Work out the finished part from the listing and answer in its coordinate system (mm). A direction names the side the tool comes from. Round coordinates to 2 decimals unless told otherwise and drop trailing zeros. Loops run counter-clockwise (first coordinate to the right, second up) from the corner with the lowest first, then second, coordinate; pieces in that order, holes last. Notation, with made-up numbers: (81.25, 74) -> (121.25, 74) arc R19 cw to (121.25, 82) -> close; hole circle Ø6 at (-2.5, 22). An arc over 180 degrees is marked (long way). Use one line per item in the form item = value.
```python
from build123d import *

# Parameters (mm, degrees)
BOSS_EXTRUDE1_DEPTH = 2
SKETCH2_W           = 40.18
SKETCH2_H           = 12.8
CUT_EXTRUDE1_DEPTH  = 1
SKETCH3_W           = 38.18
SKETCH3_H           = 10.8
CUT_EXTRUDE4_DEPTH  = 3
SKETCH4_W           = 2
SKETCH4_H           = 2
CUT_EXTRUDE5_DEPTH  = 3
SKETCH5_R           = 4
CUT_EXTRUDE6_DEPTH  = 5
SKETCH7_W           = 40.18
SKETCH7_H           = 2
BOSS_EXTRUDE2_DEPTH = 5
CUT_EXTRUDE10_DEPTH = 1
SKETCH12_W          = 40
SKETCH12_H          = 40
CUT_EXTRUDE11_DEPTH = 1
CUT_EXTRUDE12_REACH = 8
SKETCH13_R          = 1.75


with BuildPart() as part:
    # Sketch1 → Boss-Extrude1 (new body)
    with BuildSketch(Plane.XY):
        with BuildLine():
            Line((-70, -63.636363636), (70, -63.636363636))
            ThreePointArc((70, -63.636363636), (92.201532545, -2.475903873), (40, 36.363636364))
            Line((40, 36.363636364), (-40, 36.363636364))
            ThreePointArc((-40, 36.363636364), (-92.201532545, -2.475903873), (-70, -63.636363636))
        make_face()
    extrude(amount=BOSS_EXTRUDE1_DEPTH)

    # Sketch2 → Cut-Extrude1 (cut)
    with BuildSketch(Plane.XY):
        with Locations((0, 14.564946817)):
            Rectangle(SKETCH2_W, SKETCH2_H)
    extrude(amount=CUT_EXTRUDE1_DEPTH, mode=Mode.SUBTRACT)

    # Sketch3 → Cut-Extrude4 (cut, through all)
    with BuildSketch(Plane.XY):
        with Locations((0, 14.564946817)):
            Rectangle(SKETCH3_W, SKETCH3_H)
    extrude(amount=CUT_EXTRUDE4_DEPTH, mode=Mode.SUBTRACT)

    # Sketch4 → Cut-Extrude5 (cut, through all)
    with BuildSketch(Plane.XY.offset(2)):
        with Locations((-39, 35.363636364)):
            Rectangle(SKETCH4_W, SKETCH4_H)
        with Locations((39, 35.363636364)):
            Rectangle(SKETCH4_W, SKETCH4_H)
        with Locations((-68.39388, -62.636363636)):
            Rectangle(SKETCH4_W, SKETCH4_H)
        with Locations((68.39388, -62.636363636)):
            Rectangle(SKETCH4_W, SKETCH4_H)
    extrude(amount=-CUT_EXTRUDE5_DEPTH, mode=Mode.SUBTRACT)

    # Sketch5 → Cut-Extrude6 (cut)
    with BuildSketch(Plane.XY):
        with Locations((0, -15.909090909)):
            Circle(SKETCH5_R)
        with Locations((0, -39.772727273)):
            Circle(SKETCH5_R)
        with Locations((25, -39.772727273)):
            Circle(SKETCH5_R)
        with Locations((50, -39.772727273)):
            Circle(SKETCH5_R)
        with Locations((-25, -39.772727273)):
            Circle(SKETCH5_R)
        with Locations((-50, -39.772727273)):
            Circle(SKETCH5_R)
    extrude(amount=CUT_EXTRUDE6_DEPTH, mode=Mode.SUBTRACT)

    # Sketch7 → Boss-Extrude2 (add)
    with BuildSketch(Plane(origin=(0, 0, 0), x_dir=(-1, 0, 0), z_dir=(0, 0, -1))):
        with Locations((0, 7.164946817)):
            Rectangle(SKETCH7_W, SKETCH7_H)
    extrude(amount=BOSS_EXTRUDE2_DEPTH)

    # Sketch11 → Cut-Extrude10 (cut)
    with BuildSketch(Plane(origin=(0, 0, 0), x_dir=(-1, 0, 0), z_dir=(0, 0, -1))):
        Polygon((-60, -29.772727273), (-10, -29.772727273), (-10, -5.909090909), (10, -5.909090909), (10, -29.772727273), (60, -29.772727273), (60, -49.772727273), (-60, -49.772727273), align=None)
    extrude(amount=-CUT_EXTRUDE10_DEPTH, mode=Mode.SUBTRACT)

    # Sketch12 → Cut-Extrude11 (cut)
    with BuildSketch(Plane.XY.offset(2)):
        with Locations((50, -4.772727273)):
            Rectangle(SKETCH12_W, SKETCH12_H)
    extrude(amount=-CUT_EXTRUDE11_DEPTH, mode=Mode.SUBTRACT)

    # Sketch13 → Cut-Extrude12 (cut, up to next)
    with BuildSketch(Plane.XY.offset(1), mode=Mode.PRIVATE) as cut_extrude12_sk1:
        with Locations((33, 12.227272727)):
            Circle(SKETCH13_R)
    cut_extrude12_tool1 = extrude(cut_extrude12_sk1.sketch, amount=-CUT_EXTRUDE12_REACH, mode=Mode.PRIVATE) & part.part
    add(cut_extrude12_tool1.solids().sort_by_distance((33, 12.227273, 1))[0], mode=Mode.SUBTRACT)
    # Sketch13 → Cut-Extrude12 (cut, up to next)
    with BuildSketch(Plane.XY.offset(1), mode=Mode.PRIVATE) as cut_extrude12_sk2:
        with Locations((67, 12.227272727)):
            Circle(SKETCH13_R)
    cut_extrude12_tool2 = extrude(cut_extrude12_sk2.sketch, amount=-CUT_EXTRUDE12_REACH, mode=Mode.PRIVATE) & part.part
    add(cut_extrude12_tool2.solids().sort_by_distance((67, 12.227273, 1))[0], mode=Mode.SUBTRACT)
    # Sketch13 → Cut-Extrude12 (cut, up to next)
    with BuildSketch(Plane.XY.offset(1), mode=Mode.PRIVATE) as cut_extrude12_sk3:
        with Locations((33, -21.772727273)):
            Circle(SKETCH13_R)
    cut_extrude12_tool3 = extrude(cut_extrude12_sk3.sketch, amount=-CUT_EXTRUDE12_REACH, mode=Mode.PRIVATE) & part.part
    add(cut_extrude12_tool3.solids().sort_by_distance((33, -21.772727, 1))[0], mode=Mode.SUBTRACT)
    # Sketch13 → Cut-Extrude12 (cut, up to next)
    with BuildSketch(Plane.XY.offset(1), mode=Mode.PRIVATE) as cut_extrude12_sk4:
        with Locations((67, -21.772727273)):
            Circle(SKETCH13_R)
    cut_extrude12_tool4 = extrude(cut_extrude12_sk4.sketch, amount=-CUT_EXTRUDE12_REACH, mode=Mode.PRIVATE) & part.part
    add(cut_extrude12_tool4.solids().sort_by_distance((67, -21.772727, 1))[0], mode=Mode.SUBTRACT)
    # Sketch13 → Cut-Extrude12 (cut, up to next)
    with BuildSketch(Plane.XY.offset(1), mode=Mode.PRIVATE) as cut_extrude12_sk5:
        with BuildLine():
            Line((30, 9.227272727), (30, -18.772727273))
            Line((30, -18.772727273), (33, -18.772727273))
            ThreePointArc((33, -18.772727273), (35.121320344, -19.651406929), (36, -21.772727273))
            Line((36, -21.772727273), (36, -24.772727273))
            Line((36, -24.772727273), (64, -24.772727273))
            Line((64, -24.772727273), (64, -21.772727273))
            ThreePointArc((64, -21.772727273), (64.878679656, -19.651406929), (67, -18.772727273))
            Line((67, -18.772727273), (70, -18.772727273))
            Line((70, -18.772727273), (70, 9.227272727))
            Line((70, 9.227272727), (67, 9.227272727))
            ThreePointArc((67, 9.227272727), (64.878679656, 10.105952384), (64, 12.227272727))
            Line((64, 12.227272727), (64, 15.227272727))
            Line((64, 15.227272727), (36, 15.227272727))
            Line((36, 15.227272727), (36, 12.227272727))
            ThreePointArc((36, 12.227272727), (35.121320344, 10.105952384), (33, 9.227272727))
            Line((33, 9.227272727), (30, 9.227272727))
        make_face()
    cut_extrude12_tool5 = extrude(cut_extrude12_sk5.sketch, amount=-CUT_EXTRUDE12_REACH, mode=Mode.PRIVATE) & part.part
    add(cut_extrude12_tool5.solids().sort_by_distance((50, -4.772727, 1))[0], mode=Mode.SUBTRACT)


solid = part.part
```
(1) For a pull along Y with two mould halves and no side action, classify faces 1 (the flat face through (-22, -13, 0)), 2 (the flat face through (0, 6.165, -2)), 3 (the cylindrical face through (47.05, -37.07, 1.49)), 4 (the cylindrical face through (24.479, -35.807, 1.493)) as +Y half, -Y half, draft (parallel to the pull), parting line (faces both ways), or undercut.
Completed:
face_1 = draft
face_2 = -Y half
face_3 = undercut
face_4 = undercut
(2) Find section D-D, the plane z = -3.75. Write down the section's boundary in (x, y).
Completed:
outline = (-20.09, 6.16) -> (20.09, 6.16) -> (20.09, 8.16) -> (-20.09, 8.16) -> close
(3) Find section B-B, the plane x = 50. Write down the section's boundary in (y, z).
Completed:
outline = (-63.64, 0) -> (-49.77, 0) -> (-49.77, 1) -> (-43.77, 1) -> (-43.77, 2) -> (-63.64, 2) -> close; (-35.77, 1) -> (-29.77, 1) -> (-29.77, 0) -> (-24.77, 0) -> (-24.77, 2) -> (-35.77, 2) -> close; (15.23, 0) -> (35.44, 0) -> (35.44, 2) -> (15.23, 2) -> close
(4) Consider L1, parallel to Y at x = 0, z = 1.3; L2, parallel to Y at x = 33, z = 0.25; L3, parallel to X at y = -18.5, z = 0.5. Determine where each line is inside the solid, lowest interval first.
Completed:
L1 = -63.64 to -43.77, -35.77 to -19.91, -11.91 to 9.16, 19.96 to 36.36
L2 = -63.64 to -49.77, -29.77 to -23.52, -20.02 to -18.77, 9.23 to 10.48, 13.98 to 36.36
L3 = -94.5 to -10, 10 to 30, 70 to 94.5
(5) For faces 5 (the flat face through (0, 8.165, -2)), 6 (the cylindrical face through (-52.95, -37.07, 1.49)), 7 (the flat face through (31.6, -23.1, 1)), determine the directions among +Z, -Z, +X, -X, +Y, -Y from which every point of the face is accessible in a straight line to the end or side of a thin tool.
Completed:
face_5 = -Z
face_6 = +Z, -Z
face_7 = +Z
(6) Find section A-A, the plane x = 0. Write down the section's boundary in (y, z), then the cut area to 3 significant figures.
Completed:
outline = (-63.64, 0) -> (-49.77, 0) -> (-49.77, 1) -> (-43.77, 1) -> (-43.77, 2) -> (-63.64, 2) -> close; (-35.77, 1) -> (-19.91, 1) -> (-19.91, 2) -> (-35.77, 2) -> close; (-11.91, 1) -> (-5.91, 1) -> (-5.91, 0) -> (6.16, 0) -> (6.16, -5) -> (8.16, -5) -> (8.16, 1) -> (9.16, 1) -> (9.16, 2) -> (-11.91, 2) -> close; (19.96, 1) -> (20.96, 1) -> (20.96, 0) -> (36.36, 0) -> (36.36, 2) -> (19.96, 2) -> close
area = 127 mm2
(7) Given P1, Ø0.6, axis at y = 4.5, z = 1, coming from the -X side; P2, Ø1, axis at y = -7.5, z = 1, coming from the +X side; P3, Ø0.6, axis at y = 7.5, z = -2.5, coming from the -X side; P4, Ø2, axis at x = 67, y = -21.77, coming from the -Z side, each flat-ended and moving along its own axis, determine where each tip first touches the part or whether it passes through.
Completed:
P1 = -89.71
P2 = 93.55
P3 = -20.09
P4 = through
(8) Find section C-C, the plane x = 25. Write down the section's boundary in (y, z), then the cut area to 3 significant figures.
Completed:
outline = (-63.64, 0) -> (-49.77, 0) -> (-49.77, 1) -> (-43.77, 1) -> (-43.77, 2) -> (-63.64, 2) -> close; (-35.77, 1) -> (-29.77, 1) -> (-29.77, 0) -> (36.36, 0) -> (36.36, 2) -> (-35.77, 2) -> close
area = 172 mm2
